Autodesk Inventor part; units mm, degrees
ref_plane "YZ Plane" through (0, 0, 0) normal (1, 0, 0) x (0, 1, 0)
ref_plane "XZ Plane" through (0, 0, 0) normal (0, 1, 0) x (-1, 0, 0)
ref_plane "XY Plane" through (0, 0, 0) normal (0, 0, 1) x (1, 0, 0)
sketch "Sketch1" plane through (0, 0, 0) normal (0, 1, 0) x (-1, 0, 0)
  line L0 (0, 20) -> (0, -20) construction
  line L1 (-7.5, 20) -> (-7.5, -20)
  line L2 (7.5, -20) -> (7.5, 20)
  arc A0 (7.5, 20) -> (-7.5, 20) centre (0, 20) ccw
  arc A1 (-7.5, -20) -> (7.5, -20) centre (0, -20) ccw
  line L3 (0, 0) -> (40, 0) construction
  circle A2 centre (0, -20) radius 3
  circle A3 centre (0, 20) radius 3
  dimension "d1" = 20
  dimension "d2" = 90
  dimension "d3" = 15
  dimension "d4" = 6
  dimension "d5" = 6
extrude "Extrusion1" add sketch "Sketch1" along normal blind 4
properties part number "Cable_Guide_Holder_Block"
Could you check a few things on this model? Use its own coordinates, in mm. Give positions to 0.01 mm unless a question says otherwise; leave off trailing zeros. Order: outer loops, then holes, each group sorted by start corner. A loop starts at its lowest first (then second) coordinate and runs counter-clockwise, first axis right, second up. Notation, with made-up numbers: (-1, -6.75) -> (52, -6.75) arc R18 cw to (52, 18.25) -> close; hole circle Ø1 at (8, 23). An arc over 180 degrees is marked (long way). Return JSON: item names as keys, results as strings.
1. Imagine slicing it at A-A on x = 0. List the corners of the cut face in (y, z) for me, then the cut area to 3 significant figures.
Answer list:
{"outline": "(0, -27.5) -> (4, -27.5) -> (4, -23) -> (0, -23) -> close; (0, -17) -> (4, -17) -> (4, 17) -> (0, 17) -> close; (0, 23) -> (4, 23) -> (4, 27.5) -> (0, 27.5) -> close", "area": "172 mm2"}
2. Imagine slicing it at C-C on x = 4.5. List the corners of the cut face in (y, z) for me, then the cut area to 3 significant figures.
Answer list:
{"outline": "(0, -26) -> (4, -26) -> (4, 26) -> (0, 26) -> close", "area": "208 mm2"}
3. Imagine slicing it at B-B on y = 1.2. List the corners of the cut face in (x, z) for me, then the cut area to 3 significant figures.
Answer list:
{"outline": "(-7.5, -20) arc R7.5 ccw to (7.5, -20) -> (7.5, 20) arc R7.5 ccw to (-7.5, 20) -> close; hole circle Ø6 at (0, -20); hole circle Ø6 at (0, 20)", "area": "720 mm2"}
4. For pin 1 Ø1 at (x, y) = (4.5, 1) entering from +Z, with a flat end and sliding along its axis, tell me the tip position at first contact or that it passes through.
Answer list:
{"pin 1": "stops at z = 26.34"}
5. Imagine slicing it at D-D on z = 24. List the corners of the cut face in (x, y) for me.
Answer list:
{"outline": "(-6.34, 0) -> (6.34, 0) -> (6.34, 4) -> (-6.34, 4) -> close"}
6. Thinking about a two-plate mould opening in X: for faces 1 (the cylindrical face through (0.65, 1.97, 22.93)), 2 (the cylindrical face through (0.16, 1.97, 27.5)), 3 (the flat face through (7.5, 2, 0)), 4 (the cylindrical face through (0.65, 1.97, -17.07)), which applies, pulls with the +X half, pulls with the -X half, needs draft (parallel to the pull), parting line crosses it, or undercut?
Answer list:
{"face 1": "undercut", "face 2": "parting line crosses it", "face 3": "pulls with the +X half", "face 4": "undercut"}
7. I need wall thicknesses on line 1 (Z direction, x = 0, y = 1.7); line 2 (Z direction, x = 1, y = 1); line 3 (X direction, y = 1, z = 22). Which ranges of each line are inside material? Lowest first, please. Write a range as from..to.
Answer list:
{"line 1": "z = -27.5..-23, -17..17, 23..27.5", "line 2": "z = -27.43..-22.83, -17.17..17.17, 22.83..27.43", "line 3": "x = -7.23..-2.24, 2.24..7.23"}
